```python
from build123d import *

# Parameters (mm, degrees)
F0_W           = 203.2
F0_H           = 203.2
F1_DEPTH       = 101.6
F3_D           = 26.9748
F3_CSINK_D     = 49.2252
F3_CSINK_ANGLE = 82
F5_D           = 26.9748
F5_CSINK_D     = 49.2252
F5_CSINK_ANGLE = 82


with BuildPart() as f1:
    # F0 (on Front) → F1 (new body, symmetric)
    with BuildSketch(Plane.XZ):
        with Locations((-101.6, 101.6)):
            Rectangle(F0_W, F0_H)
    extrude(amount=F1_DEPTH, both=True)

    # F3 (through all)
    with Locations(Plane.XZ.offset(101.6)):
        with Locations((-56.698719, 146.501281), (-146.501281, 146.501281), (-146.501281, 56.698719), (-56.698719, 56.698719)):
            CounterSinkHole(F3_D / 2, F3_CSINK_D / 2, counter_sink_angle=F3_CSINK_ANGLE)

    # F5 (through all)
    with Locations(Plane.XY.offset(203.2)):
        with Locations((-56.698719, 44.901281), (-146.501281, 44.901281), (-146.501281, -44.901281), (-56.698719, -44.901281)):
            CounterSinkHole(F5_D / 2, F5_CSINK_D / 2, counter_sink_angle=F5_CSINK_ANGLE)


solid = f1.part
```
The listing builds one solid part. Answer for the finished solid, in the listing's coordinates (mm). Coordinates: 2 decimals unless noted, no trailing zeros. Loops run counter-clockwise (first coordinate to the right, second up) from the corner with the lowest first, then second, coordinate; pieces in that order, holes last. Notation, with made-up numbers: M 81.5,74.5 L 87.5,74.5 A26 ccw 87.5,93.5 Z; hole C -10.5,-31.5 d11. An arc over 180 degrees is marked long. Answer as a JSON object with one key per item and string values. Group by question number.
Item 1: Section C-C (z = 138) is taken. Give the number of separate pieces and of enclosed holes in the cut face, and give its area (3 significant figures).
Item 2: Section B-B (y = 88.5) is taken. Write down the section's boundary in (x, z), and give its area (3 significant figures).
Item 3: Section A-A (z = 176) is taken. Write down the section's boundary in (x, y).
Item 4: Consider L1, parallel to X at y = 52, z = 69.5; L2, parallel to X at y = -40.5, z = 86; L3, parallel to Z at x = -153.5, y = -4.5. Determine where each line is inside the solid, lowest interval first.
Item 5: Determine the mould class of faces 1 (the face through (-43.224, 79.947, 57.292)), 2 (the face through (-159.366, -40.85, 100.971)), 3 (the face through (-70.079, -40.688, 191.023)) for opening direction Z: +Z half, -Z half, draft (parallel to the pull), parting line (faces both ways), or undercut.
Item 6: This flat-tipped pin is pushed along its axis until it touches: P1, Ø24.5, axis at x = -56.7, y = 44.9, coming from the +Z side. Where does it stop, or does it pass through?
Solved:
{
 "1": {"separate pieces": "3", "enclosed holes": "0", "area": "32,200 mm2"},
 "2": {"outline": "M -203.2,0 L 0,0 L 0,203.2 L -203.2,203.2 Z; hole C -146.5,56.7 d26.97; hole C -146.5,146.5 d26.97; hole C -56.7,56.7 d26.97; hole C -56.7,146.5 d26.97", "area": "39,000 mm2"},
 "3": {"outline": "M -203.2,-101.6 L 0,-101.6 L 0,101.6 L -203.2,101.6 Z; hole C -146.5,-44.9 d26.97; hole C -146.5,44.9 d26.97; hole C -56.7,-44.9 d26.97; hole C -56.7,44.9 d26.97"},
 "4": {"L1": "x = -203.2 to -157.97, -135.03 to -68.17, -45.23 to 0", "L2": "x = -203.2 to -159.25, -133.75 to -69.45, -43.95 to 0", "L3": "z = 0 to 45.17, 68.23 to 134.97, 158.03 to 203.2"},
 "5": {"face 1": "undercut", "face 2": "draft", "face 3": "+Z half"},
 "6": {"P1": "passes through"}
}
